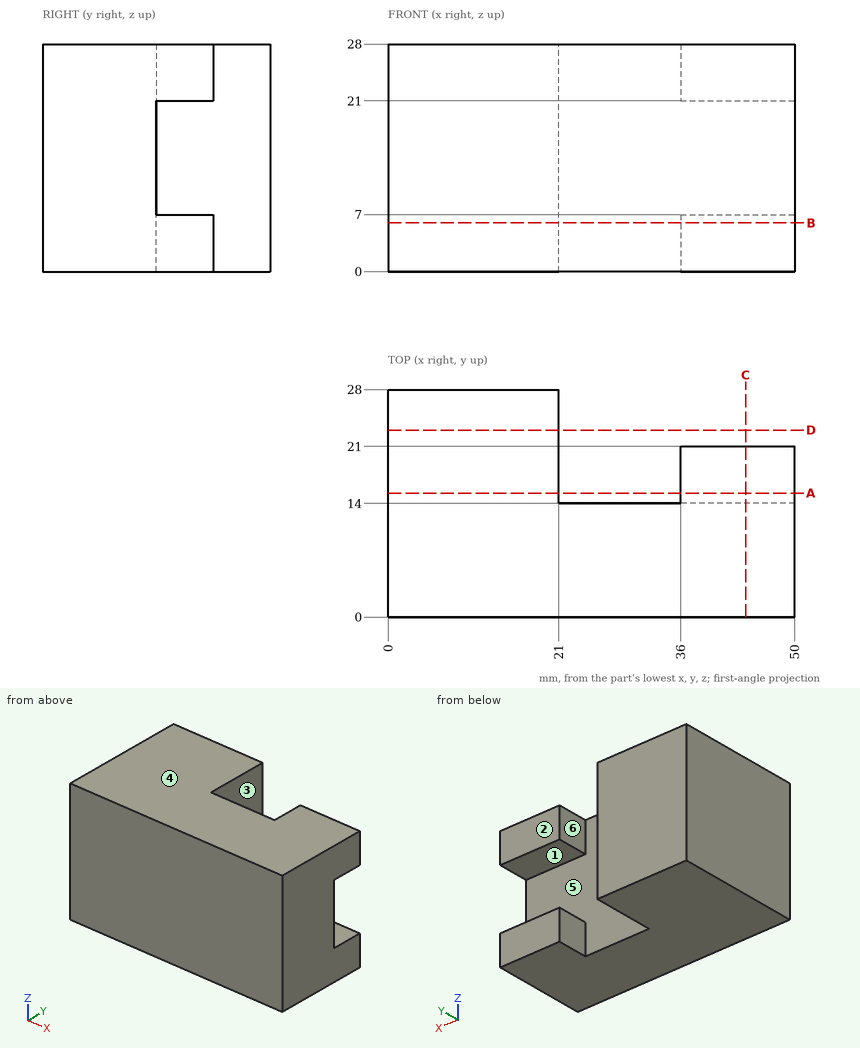
The drawing under review shows one solid part. Ordinate dimensions are in mm from its lowest x, y, z. A direction names the side the tool comes from. Coordinates: 2 decimals unless noted, no trailing zeros. Write each loop counter-clockwise with the first axis right and the second up, starting at its lowest first coordinate (ties: lowest second). Pieces come first, ordered by that corner, then holes.
1) Machinability: for the marked faces 1, 2 and 3, which of the approach directions +Z, -Z, +X, -X, +Y, -Y give a long, thin tool a straight path to every point of the face, cutting with its end or side? Answer none if there is none.
2) Add section D-D (y = 23). Write out the cut boundary in (x, z).
3) Mouldability with a two-part tool opening along Z and no side actions: class the marked faces 4, 5 and 6 as +Z half, -Z half, draft (parallel to the pull), parting line (faces both ways), or undercut.
4) To check wall thickness, follow L1, parallel to X at y = 14.25, z = 25.25; L2, parallel to Y at x = 22, z = 20.5; L3, parallel to X at y = 26.5, z = 22.5. State the ranges of each line that lie inside material, in increasing order.
5) Insertion check: pin 1 (3.5 mm diameter, centred on x = 45.5, z = 25.5, fed in from +Y); pin 2 (1 mm diameter, centred on x = 37.5, z = 13, fed in from +Y). Each pin has a flat end and moves straight along its axis. Give the tip position at first contact, or say it passes through.
6) Add section A-A (y = 15.25). Write out the cut boundary in (x, z), plus the area to 3 significant figures.
7) Add section C-C (x = 44). Write out the cut boundary in (y, z), plus the area to 3 significant figures.
8) Add section B-B (z = 6). Write out the cut boundary in (x, y).
Check result:
1. face 1: +X, +Y
1. face 2: +Z, -Z, +X, +Y
1. face 3: +Z, -Z, +Y
2. outline: (0, 0) - (21, 0) - (21, 28) - (0, 28) - close
3. face 4: +Z half
3. face 5: undercut
3. face 6: draft
4. L1: x = 0 to 21, 36 to 50
4. L2: y = 0 to 14
4. L3: x = 0 to 21
5. pin 1: stops at y = 21
5. pin 2: stops at y = 14
6. outline: (0, 0) - (21, 0) - (21, 28) - (0, 28) - close; (36, 0) - (50, 0) - (50, 7) - (36, 7) - close; (36, 21) - (50, 21) - (50, 28) - (36, 28) - close
6. area: 784 mm2
7. outline: (0, 0) - (21, 0) - (21, 7) - (14, 7) - (14, 21) - (21, 21) - (21, 28) - (0, 28) - close
7. area: 490 mm2
8. outline: (0, 0) - (50, 0) - (50, 21) - (36, 21) - (36, 14) - (21, 14) - (21, 28) - (0, 28) - close
